```python
from build123d import *

# Parameters (mm, degrees)
PAD009_DEPTH         = 10
PAD010_DEPTH         = 10
POCKET011_DEPTH      = 223.4231860076
SKETCH024_R          = 15
SKETCH024_R_2        = 1.5
SKETCH024_R_3        = 2
POCKET012_DEPTH      = 10.001
POCKET012_DEPTH_BACK = 10.001
POCKET013_DEPTH      = 3


with BuildPart() as part:
    # Sketch021 → Pad009 (new body)
    with BuildSketch(Plane.XY.offset(40.1)):
        with BuildLine():
            Line((-25.5, 27.5), (25.5, 27.5))
            ThreePointArc((27.5, 25.5), (26.9142135624, 26.9142135624), (25.5, 27.5))
            Line((27.5, 25.5), (27.5, -25.5))
            ThreePointArc((25.5, -27.5), (26.9142135624, -26.9142135624), (27.5, -25.5))
            Line((25.5, -27.5), (-25.5, -27.5))
            ThreePointArc((-27.5, -25.5), (-26.9142135624, -26.9142135624), (-25.5, -27.5))
            Line((-27.5, -25.5), (-27.5, 25.5))
            ThreePointArc((-25.5, 27.5), (-26.9142135624, 26.9142135624), (-27.5, 25.5))
        make_face()
    extrude(amount=PAD009_DEPTH)

    # Sketch022 → Pad010 (join)
    with BuildSketch(Plane.XY.offset(50.1)):
        with BuildLine():
            Line((-27.5, 0), (-22.5, 0))
            Line((-22.5, 0), (-22.5, -5))
            Line((-22.5, -5), (-15.1966113671, -8.26504433))
            ThreePointArc((-15.1966113671, -8.26504433), (0, -19.2587479987), (15.1966113671, -8.26504433))
            Line((22.5, -5), (15.1966113671, -8.26504433))
            Line((22.5, 0), (22.5, -5))
            Line((22.5, 0), (27.5, 0))
            Line((27.5, -16.7), (27.5, 0))
            Line((19, -20.5), (27.5, -16.7))
            Line((19, -27.5), (19, -20.5))
            Line((-19, -27.5), (19, -27.5))
            Line((-19, -20.5), (-19, -27.5))
            Line((-27.5, -16.7), (-19, -20.5))
            Line((-27.5, 0), (-27.5, -16.7))
        make_face()
    extrude(amount=PAD010_DEPTH)

    # Sketch023 (on Face25 of Pad010) → Pocket011 (cut, through all)
    with BuildSketch(Plane(origin=(-10.8029761218, -24.1645518514, 0), x_dir=(0.9129235791, -0.4081305413, 0), z_dir=(-0.4081305413, -0.9129235791, 0))):
        with BuildLine():
            Line((-15.6342451471, 60.1), (-11.6342451471, 60.1))
            Line((-11.6342451471, 60.1), (-11.6342451471, 54.1))
            ThreePointArc((-15.6342451471, 54.1), (-13.6342451471, 52.1), (-11.6342451471, 54.1))
            Line((-15.6342451471, 60.1), (-15.6342451471, 54.1))
        make_face()
    pocket011 = extrude(amount=-POCKET011_DEPTH, mode=Mode.SUBTRACT)

    # Mirrored: Pocket011 across YZ
    add(pocket011.mirror(Plane.YZ), mode=Mode.SUBTRACT)

    # Sketch024 → Pocket012 (cut, two sides)
    with BuildSketch(Plane.XY.offset(50.1)) as pocket012_sk:
        Circle(SKETCH024_R)
        with Locations((15.495, 15.495)):
            Circle(SKETCH024_R_2)
        with Locations((15.495, -15.495)):
            Circle(SKETCH024_R_2)
        with Locations((-15.495, -15.495)):
            Circle(SKETCH024_R_2)
        with Locations((-15.495, 15.495)):
            Circle(SKETCH024_R_2)
        with Locations((-19.5, 19.5)):
            Circle(SKETCH024_R_3)
        with Locations((-13.5, -19.5)):
            Circle(SKETCH024_R_3)
        with Locations((13.5, -19.5)):
            Circle(SKETCH024_R_3)
        with Locations((19.5, 19.5)):
            Circle(SKETCH024_R_3)
    extrude(amount=-POCKET012_DEPTH, mode=Mode.SUBTRACT)
    extrude(pocket012_sk.sketch, amount=POCKET012_DEPTH_BACK, mode=Mode.SUBTRACT)

    # Sketch026 → Pocket013 (cut)
    with BuildSketch(Plane.XY.offset(40.1)):
        Polygon((22.9641016151, 17.5), (22.9641016151, 21.5), (19.5, 23.5), (16.0358983849, 21.5), (16.0358983849, 17.5), (19.5, 15.5), align=None)
        Polygon((16.9641016151, -21.5), (16.9641016151, -17.5), (13.5, -15.5), (10.0358983849, -17.5), (10.0358983849, -21.5), (13.5, -23.5), align=None)
        Polygon((-10.0358983849, -21.5), (-10.0358983849, -17.5), (-13.5, -15.5), (-16.9641016151, -17.5), (-16.9641016151, -21.5), (-13.5, -23.5), align=None)
        Polygon((-16.0358983849, 17.5), (-16.0358983849, 21.5), (-19.5, 23.5), (-22.9641016151, 21.5), (-22.9641016151, 17.5), (-19.5, 15.5), align=None)
    extrude(amount=POCKET013_DEPTH, mode=Mode.SUBTRACT)


solid = part.part
```
Design review of the part built by this model. Coordinates are the model's own, in mm. A direction names the side the tool comes from. Round coordinates to 2 decimals unless told otherwise and drop trailing zeros. Write each loop counter-clockwise with the first axis right and the second up, starting at its lowest first coordinate (ties: lowest second). Pieces come first, ordered by that corner, then holes. Notation, with made-up numbers: (-40, 44.25) -> (-23, 44.25) arc R7 cw to (-23, 53.25) -> close; hole circle Ø9 at (-23, 7.25). An arc over 180 degrees is marked (long way). Answer in a Markdown table with one row per item.
Q1. Clearance check with flat-ended pins moving along their axes: pin 1 Ø4 at (x, z) = (-25, 55.5) entering from +Y; pin 2 Ø2.5 at (x, y) = (25, -22) entering from +Z; pin 3 Ø3.5 at (x, y) = (13, -19) entering from -Z. State where each tip first meets the part, or that it passes through.
The answers:
| item | result |
|---|---|
| pin 1 | y = 0 |
| pin 2 | z = 50.1 |
| pin 3 | z = 43.1 |
Q2. To check wall thickness, follow L1, parallel to X at y = -19.5, z = 54.25; L2, parallel to X at y = -18.5, z = 48.75; L3, parallel to X at y = -12.5, z = 57.5. State the ranges of each line that lie inside material, in increasing order. Write a range as [from, to].
The answers:
| item | result |
|---|---|
| L1 | [-21.24, -15.5], [-11.5, 11.5], [15.5, 21.24] |
| L2 | [-27.5, -15.23], [-11.77, 11.77], [15.23, 27.5] |
| L3 | [-27.5, -22.71], [-18.33, -13.06], [13.06, 18.33], [22.71, 27.5] |
Q3. Take a section at B-B, the plane y = 19.5. State the section outline as (x, z) points.
The answers:
| item | result |
|---|---|
| outline | (-27.5, 40.1) -> (-22.96, 40.1) -> (-22.96, 43.1) -> (-21.5, 43.1) -> (-21.5, 50.1) -> (-27.5, 50.1) -> close; (-17.5, 43.1) -> (-16.04, 43.1) -> (-16.04, 40.1) -> (16.04, 40.1) -> (16.04, 43.1) -> (17.5, 43.1) -> (17.5, 50.1) -> (-17.5, 50.1) -> close; (21.5, 43.1) -> (22.96, 43.1) -> (22.96, 40.1) -> (27.5, 40.1) -> (27.5, 50.1) -> (21.5, 50.1) -> close |
Q4. Take a section at C-C, the plane z = 58.75. State the section outline as (x, y) points (3 decimals), then the cut area to 3 significant figures.
The answers:
| item | result |
|---|---|
| outline | (-27.5, -16.7) -> (-25.076, -17.784) -> (-19.884, -6.17) -> (-22.5, -5) -> (-22.5, 0) -> (-27.5, 0) -> close; (-21.424, -19.416) -> (-19, -20.5) -> (-19, -27.5) -> (19, -27.5) -> (19, -20.5) -> (21.424, -19.416) -> (16.232, -7.802) -> (15.197, -8.265) arc R16 cw to (-15.197, -8.265) -> (-16.232, -7.802) -> close; (19.884, -6.17) -> (25.076, -17.784) -> (27.5, -16.7) -> (27.5, 0) -> (22.5, 0) -> (22.5, -5) -> close; hole circle Ø3 at (-15.495, -15.495); hole circle Ø4 at (-13.5, -19.5); hole circle Ø4 at (13.5, -19.5); hole circle Ø3 at (15.495, -15.495) |
| area | 627 mm² |
Q5. Draft analysis for pull direction X (two halves, no side actions). For faces 1 (the face through (-26.9, 26.93, 45.03)), 2 (the face through (-21.256, 16.514, 41.579)), 3 (the face through (13, 13, 40.1)), state which applies: +X half, -X half, draft (parallel to the pull), parting line (faces both ways), or undercut.
The answers:
| item | result |
|---|---|
| face 1 | -X half |
| face 2 | undercut |
| face 3 | draft |
Q6. Take a section at A-A, the plane x = 0. State the section outline as (y, z) points.
The answers:
| item | result |
|---|---|
| outline | (-27.5, 40.1) -> (-15, 40.1) -> (-15, 50.1) -> (-19.26, 50.1) -> (-19.26, 60.1) -> (-27.5, 60.1) -> close; (15, 40.1) -> (27.5, 40.1) -> (27.5, 50.1) -> (15, 50.1) -> close |
Q7. Take a section at D-D, the plane y = 5. State the section outline as (x, z) points, then the cut area to 3 significant figures.
The answers:
| item | result |
|---|---|
| outline | (-27.5, 40.1) -> (-14.14, 40.1) -> (-14.14, 50.1) -> (-27.5, 50.1) -> close; (14.14, 40.1) -> (27.5, 40.1) -> (27.5, 50.1) -> (14.14, 50.1) -> close |
| area | 267 mm² |
Q8. For faces 4 (the face through (25, 0, 55)), 5 (the face through (-19, -24, 55)), 6 (the face through (17.792, 22.514, 41.579)), list the 3-axis set-ups (+Z, -Z, +X, -X, +Y, -Y) from which the entire face can be reached by the end or side of a thin tool; tool diameter is ignored.
The answers:
| item | result |
|---|---|
| face 4 | +Z, +X, -X, +Y |
| face 5 | +Z, -X, -Y |
| face 6 | -Z |
